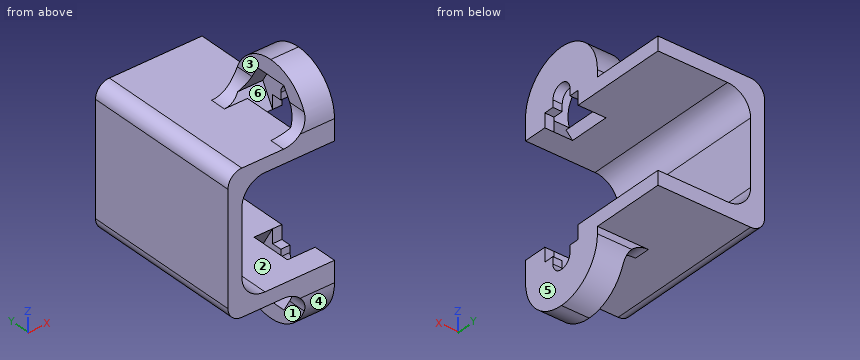
Autodesk Inventor part; units mm, degrees
ref_plane "YZ Plane" through (0, 0, 0) normal (1, 0, 0) x (0, 1, 0)
ref_plane "XZ Plane" through (0, 0, 0) normal (0, 1, 0) x (-1, 0, 0)
ref_plane "XY Plane" through (0, 0, 0) normal (0, 0, 1) x (1, 0, 0)
sketch "Sketch1" plane through (0, 0, 0) normal (0, 1, 0) x (-1, 0, 0)
  line L0 (0, 0) -> (0, -1.5)
  line L1 (0, -1.5) -> (10, -1.5)
  line L2 (10, -1.5) -> (10, -13.5)
  line L3 (10, -13.5) -> (0, -13.5)
  line L4 (0, -13.5) -> (0, -15)
  line L5 (0, -15) -> (11.5, -15)
  line L6 (11.5, -15) -> (11.5, 0)
  line L7 (11.5, 0) -> (0, 0)
  dimension "d0" = 1.5
  dimension "d1" = 1.5
  dimension "d2" = 1.5
  dimension "d3" = 10
  dimension "d4" = 12
extrude "Extrusion1" add sketch "Sketch1" along normal blind 17.5
fillet "Fillet1" radius 1.5 2 edges at (-11.5, 8.75, 0) (-11.5, 8.75, -15)
fillet "Fillet2" radius 2.5 2 edges at (-10, 8.75, -13.5) (-10, 8.75, -1.5)
sketch "Sketch2" plane through (0, 0, 0) normal (0, -1, 0) x (1, 0, 0)
  line L0 (0, 0) -> (-3, 0)
  line L1 (-3, 0) -> (-3, 5.5)
  line L2 (-3, 5.5) -> (0, 5.5)
  line L3 (0, 5.5) -> (0, 0)
  line L4 (0, -15) -> (-10, -15)
  line L5 (0, -15) -> (-3, -15)
  line L6 (-3, -15) -> (-3, -20.5)
  line L7 (-3, -20.5) -> (0, -20.5)
  line L8 (0, -20.5) -> (0, -15)
  dimension "d9" = 3
  dimension "d10" = 5.5
extrude "Extrusion2" add sketch "Sketch2" against normal blind 9.5
fillet "Fillet3" radius 4.75 4 edges at (-1.5, 0, 5.5) (-1.5, 9.5, 5.5) (-1.5, 0, -20.5) (-1.5, 9.5, -20.5)
fillet "Fillet4" radius 2.5 2 edges at (-3, 4.75, -15) (-3, 4.75, 0)
sketch "Sketch3" plane through (-3, 4.75, -15.75) normal (-1, 0, 0) x (0, 0, 1)
  arc A0 (0, 4.75) -> (0, -4.75) centre (0, 0) ccw
  circle A1 centre (0, 0) radius 3.5
  line L0 (-3.0311, -1.75) -> (-3.0311, 1.75)
  line L1 (-3.0311, 1.75) -> (0, 3.5)
  line L2 (0, 3.5) -> (3.0311, 1.75)
  line L3 (3.0311, 1.75) -> (3.0311, -1.75)
  line L4 (3.0311, -1.75) -> (0, -3.5)
  line L5 (0, -3.5) -> (-3.0311, -1.75)
  line L6 (2.25, -4.75) -> (2.25, 12.75)
  circle A2 centre (0, 0) radius 1.125
  line L7 (0.75, -4.75) -> (0.75, 4.75)
  line L8 (0.75, 3.067) -> (0.75, -3.067)
  arc A3 (18.25, -4.4159) -> (18.25, 4.4159) centre (16.5, 0) ccw
  line L9 (19.5311, 1.75) -> (19.5311, -1.75)
  line L10 (19.5311, -1.75) -> (16.5, -3.5)
  line L11 (16.5, -3.5) -> (13.4689, -1.75)
  line L12 (13.4689, -1.75) -> (13.4689, 1.75)
  line L13 (13.4689, 1.75) -> (16.5, 3.5)
  line L14 (16.5, 3.5) -> (19.5311, 1.75)
  line L15 (14.25, 12.75) -> (14.25, -4.75)
  line L16 (15.75, -4.75) -> (15.75, 12.75)
  line L17 (15.75, -3.067) -> (15.75, 3.067)
  circle A4 centre (16.5, 0) radius 1.125
  point P0 (2.25, -2.201)
  point P1 (2.25, 2.201)
  point P2 (0.75, 0.8385)
  point P3 (0.75, -0.8385)
  point P4 (15.75, 0.8385)
  point P5 (15.75, -0.8385)
  point P6 (14.25, 2.201)
  point P7 (14.25, -2.201)
  dimension "d15" = 3.5
  dimension "d16" = 2.25
  dimension "d25" = 2.25
extrude "Extrusion3" cut sketch "Sketch3" along normal blind 10 and the other way blind 2 contours L7 A2 L4 L5 L0 L1 L2 | L7 A2 | L9 L10 L11 L16 A4 L13 L14 | A4 L16 picked at (0.2626, -0.3643) picked at (16.8752, 0.2073)
extrude "Extrusion4" cut sketch "Sketch3" against normal through all contours L7 A2 | A2 L7 | A4 L16 | L16 A4
extrude "Extrusion5" cut sketch "Sketch3" against normal up to surface (2 mm away) contours L6 L4 L7 A2 L2 | L16 A4 L11 L15 L13
sketch "Sketch4" plane through (0, 0, -13.5) normal (1, 0, 0) x (0, 0, -1)
  circle A0 centre (2.25, 4.75) radius 1.125
  line L0 (2.25, 5.875) -> (-14.25, 5.875)
  line L1 (-14.25, 5.875) -> (-14.25, 3.625)
  line L2 (-14.25, 3.625) -> (2.25, 3.625)
  line L3 (2.25, 3.625) -> (2.25, 5.875)
  circle A1 centre (-14.25, 4.75) radius 1.125
  point P0 (-13.5, 0)
  point P1 (2.25, 3.625)
extrude "Extrusion6" cut sketch "Sketch4" against normal up to surface (1 mm away) contours A0 L2 A1 L0
sketch "Sketch5" plane through (0, 17.5, 0) normal (1, 0, 0) x (0, 0, -1)
  line L0 (0, -17.5) -> (0, 0)
  line L1 (15, -9.683) -> (15, -15.817)
  line L2 (0, -10.549) -> (15, -10.549)
  line L3 (15, -10.549) -> (15, -14.951)
  line L4 (15, -14.951) -> (0, -14.951)
  line L5 (0, -14.951) -> (0, -10.549)
  point P0 (13.5, -14.951)
  point P1 (1.5, -10.549)
  point P2 (0, -14.951)
extrude "Extrusion7" cut sketch "Sketch5" against normal up to surface (3 mm away)
properties part number "Pololu_MicroMotorMount"
Geometry check sheet. Reference: the model listing, model coordinates, mm. Face numbers are marked on the shaded views. A direction names the side the tool comes from. Coordinates: 2 decimals unless noted, no trailing zeros. Order: outer loops, then holes, each group sorted by start corner. A loop starts at its lowest first (then second) coordinate and runs counter-clockwise, first axis right, second up. Notation, with made-up numbers: M 37,63.25 L 93,63.25 A33 cw 93,94.25 Z; hole C 26.25,43.5 d1. An arc over 180 degrees is marked long. One line per question, with ' | ' between items. Start each with the question number.
Item 1: Cross-section at C-C on y = 5.5. Enter the section's corners in (x, z).
Item 2: Cross-section at B-B on y = 16. Enter the section's corners in (x, z).
Item 3: Draft check along Y on the marked faces 4, 5 and 6. Enter one of: pulls with the +Y half, pulls with the -Y half, needs draft (parallel to the pull), parting line crosses it, or undercut.
Item 4: Set-up check for the marked faces 1, 2 and 3: record each of +Z, -Z, +X, -X, +Y, -Y from which the full face is reachable in a straight line by a thin tool's end or side.
Item 5: Material ranges on L1, parallel to Z at x = -7, y = 5; L2, parallel to X at y = 12.25, z = -4.25; L3, parallel to X at y = 5.5, z = 4, recorded low to high. Write a range as [from, to].
Item 6: Cross-section at D-D on z = -14.5. Enter the section's corners in (x, y).
Item 7: Gauge pin test, flat ends, axial feed: pin 1 (3 mm diameter, centred on x = -10.5, y = 15, fed in from -Z); pin 2 (2 mm diameter, centred on x = -5.5, y = 8.5, fed in from -Z); pin 3 (0.5 mm diameter, centred on x = -0.5, y = 3.5, fed in from -Z); pin 4 (4 mm diameter, centred on x = -6.5, z = -8, fed in from -Y). Record the tip position at first contact, or that the pin passes through.
Findings:
1) outline: M -11.5,-13.5 A1.5 ccw -10,-15 L -3,-15 L -3,-13.5 L -7.5,-13.5 A2.5 cw -10,-11 L -10,-4 A2.5 cw -7.5,-1.5 L -3,-1.5 L -3,0 L -10,0 A1.5 ccw -11.5,-1.5 Z; M -3,-20.44 L 0,-20.44 L 0,-16.59 L -1,-16.59 L -1,-18.78 L -3,-18.78 Z; M -3,3.78 L -1,3.78 L -1,1.59 L 0,1.59 L 0,5.44 L -3,5.44 Z
2) outline: M -11.5,-13.5 A1.5 ccw -10,-15 L 0,-15 L 0,-13.5 L -7.5,-13.5 A2.5 cw -10,-11 L -10,-4 A2.5 cw -7.5,-1.5 L 0,-1.5 L 0,0 L -10,0 A1.5 ccw -11.5,-1.5 Z
3) face 4: pulls with the -Y half | face 5: needs draft | face 6: undercut
4) face 1: -Z, -X, +Y, -Y | face 2: +X, +Y, -Y | face 3: +Z, -X, +Y, -Y
5) L1: z = [-15, -13.5], [-1.5, 0] | L2: x = [-11.5, -10] | L3: x = [-3, 0]
6) outline: M -11.12,0 L 0,0 L 0,2.55 L -1,2.55 L -1,1.97 L -3,1.97 L -3,7.53 L -1,7.53 L -1,6.95 L 0,6.95 L 0,17.5 L -11.12,17.5 Z
7) pin 1: stops at z = -15 | pin 2: stops at z = -15.21 | pin 3: stops at z = -20.39 | pin 4: passes through
